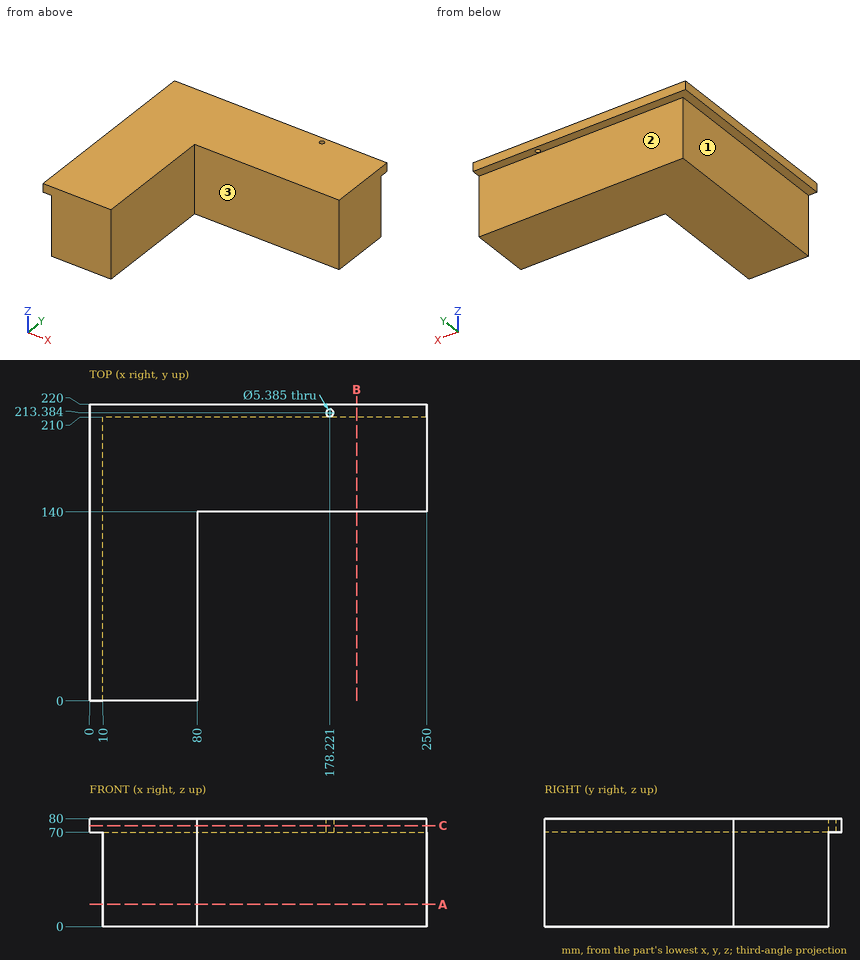
Here's the drawing with two shaded views (mm, measured from the low corner). I have some questions. A direction names the side the tool comes from. Give positions to 0.01 mm unless a question says otherwise; leave off trailing zeros. Write each loop counter-clockwise with the first axis right and the second up, starting at its lowest first coordinate (ties: lowest second). Pieces come first, ordered by that corner, then holes. Notation, with made-up numbers: (75.25, 20) -> (97.25, 20) arc R26 ccw to (97.25, 54) -> close; hole circle Ø2 at (54.5, 80). An arc over 180 degrees is marked (long way). Use one line per item in the form item = value.
1) If I drill on L1, parallel to Y at x = 171, z = 30; L2, parallel to X at y = 166.5, z = 20.5; L3, parallel to X at y = 15.5, z = 55, over which ranges is the centre line in solid material (lowest first)? Write a range as [from, to].
Verdict:
L1 = [140, 210]
L2 = [10, 250]
L3 = [10, 80]
2) On a 3-axis mill with a long thin cutter (end or side, diameter ignored), from which of +Z, -Z, +X, -X, +Y, -Y can I reach the whole of each face in a straight line? I mean the marked faces 1, 2 and 3. Say none if no direction works.
Verdict:
face_1 = -Z, -X, +Y, -Y
face_2 = -Z, +X, -X, +Y
face_3 = +Z, -Z, +X, -Y
3) Suppose I cut it at C-C (z = 75). Please give me the cut outline in (x, y) (1 decimal), and give its area (3 significant figures).
Verdict:
outline = (0, 0) -> (80, 0) -> (80, 140) -> (250, 140) -> (250, 220) -> (0, 220) -> close; hole circle Ø5.4 at (178.2, 213.4)
area = 31,200 mm2
4) Suppose I cut it at B-B (x = 198). Please give me the cut outline in (y, z).
Verdict:
outline = (140, 0) -> (210, 0) -> (210, 70) -> (220, 70) -> (220, 80) -> (140, 80) -> close
5) I'm going to push flat-ended pins straight in: pin 1 (2 mm diameter, centred on x = 191, z = 13.5, fed in from -Y); pin 2 (10 mm diameter, centred on y = 31, z = 69, fed in from +X); pin 3 (12 mm diameter, centred on y = 29, z = 13.5, fed in from -X). Where does each tip first touch, or does it pass through?
Verdict:
pin_1 = 140
pin_2 = 80
pin_3 = 10
6) Suppose I cut it at A-A (z = 16.5). Please give me the cut outline in (x, y).
Verdict:
outline = (10, 0) -> (80, 0) -> (80, 140) -> (250, 140) -> (250, 210) -> (10, 210) -> close
